Here's how the part is built. I have some questions about the finished solid (model axes, mm). Face numbers are marked on the shaded views. A direction names the side the tool comes from. Coordinates: 2 decimals unless noted, no trailing zeros. Write each loop counter-clockwise with the first axis right and the second up, starting at its lowest first coordinate (ties: lowest second). Pieces come first, ordered by that corner, then holes. Notation, with made-up numbers: M 2,-28 L 7,-28 A13 cw 7,-11 Z; hole C 85,-38.75 d6. An arc over 180 degrees is marked long. Use a Markdown table: item, result.
```python
from build123d import *

# Parameters (mm, degrees)
BOSS_EXTRUDE1_DEPTH = 30
SKETCH3_R           = 2
CUT_EXTRUDE1_DEPTH  = 49.344936653
FILLET1_R           = 2.5


with BuildPart() as part:
    # Sketch2 → Boss-Extrude1 (new, symmetric)
    with BuildSketch(Plane(origin=(0, 0, 0), x_dir=(0, 0, -1), z_dir=(1, 0, 0))):
        with BuildLine():
            Line((0, 0), (17.093183557, 0))
            ThreePointArc((17.093183557, 0), (23.540778857, 1.87930265), (27.968877001, 6.928580859))
            Line((27.968877001, 6.928580859), (32.531082361, 16.712261826))
            ThreePointArc((32.531082361, 16.712261826), (32.587511126, 16.763969262), (32.663974966, 16.760630779))
            Line((32.663974966, 16.760630779), (32.845236523, 16.676107126))
            ThreePointArc((32.845236523, 16.676107126), (33.879385242, 15.547531839), (33.812615574, 14.018255029))
            Line((33.812615574, 14.018255029), (30.053384911, 5.956558857))
            ThreePointArc((30.053384911, 5.956558857), (24.776567956, -0.060497675), (17.093183557, -2.3))
            Line((17.093183557, -2.3), (2.3, -2.3))
            Line((2.3, -2.3), (0, 0))
        make_face()
    extrude(amount=BOSS_EXTRUDE1_DEPTH, both=True)

    # Sketch3 → Cut-Extrude1 (cut, through all)
    with BuildSketch(Plane(origin=(0, 0, 0), x_dir=(1, 0, 0), z_dir=(0, 1, 0))):
        with BuildLine():
            Line((-26.9, 13.33), (-30, 13.33))
            Line((-30, 13.33), (-30, 0))
            Line((-30, 0), (-22.5, 0))
            Line((-22.5, 0), (-22.5, 8.93))
            ThreePointArc((-22.5, 8.93), (-23.788730163, 12.041269837), (-26.9, 13.33))
        make_face()
        with Locations(Location((-17, 9.5, 0), (0, 0, 270))):
            Circle(SKETCH3_R)
        with Locations(Location((17, 9.5, 0), (0, 0, 270))):
            Circle(SKETCH3_R)
        with BuildLine():
            Line((30, 0), (30, 13.33))
            Line((30, 13.33), (26.9, 13.33))
            ThreePointArc((26.9, 13.33), (23.788730163, 12.041269837), (22.5, 8.93))
            Line((22.5, 8.93), (22.5, 0))
            Line((22.5, 0), (30, 0))
        make_face()
    extrude(amount=-CUT_EXTRUDE1_DEPTH, mode=Mode.SUBTRACT)

    # Fillet1
    fillet1_edges = [part.edges().sort_by_distance(p)[0] for p in [
        (-30, -1.15, -13.33),
        (30, -1.15, -13.33),
    ]]
    fillet(fillet1_edges, radius=FILLET1_R)


solid = part.part
```
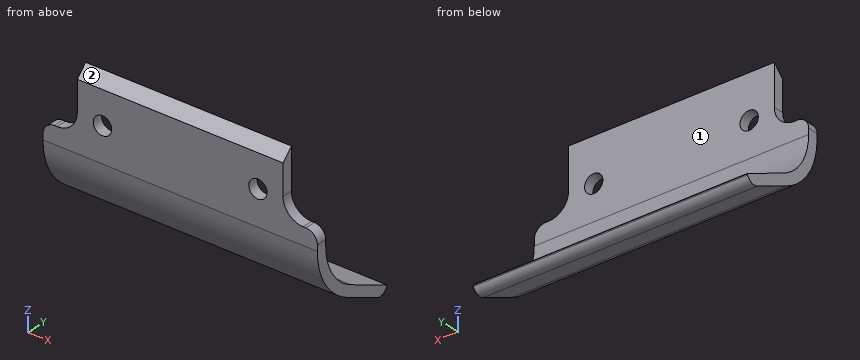
1. Suppose I cut it at A-A on x = 17. Write out the boundary of the cut face in (y, z).
Answers follow:
| item | result |
|---|---|
| outline | M -2.3,-17.09 A14.3 ccw 5.96,-30.05 L 14.02,-33.81 A2 ccw 16.68,-32.85 L 16.76,-32.66 A0.1 ccw 16.71,-32.53 L 6.93,-27.97 A12 cw 0,-17.09 L 0,-11.5 L -2.3,-11.5 Z; M -2.3,-7.5 L 0,-7.5 L 0,0 L -2.3,-2.3 Z |
2. Will these pins go through, and if not, where does the flat tip stop? pin 1 Ø8.5 at (x, z) = (-13.5, -10.5) entering from +Y; pin 2 Ø6 at (x, y) = (-15, 13.5) entering from +Z; pin 3 Ø1.8 at (y, z) = (-0.5, -2.5) entering from -X.
Answers follow:
| item | result |
|---|---|
| pin 1 | stops at y = 0 |
| pin 2 | stops at z = -29.63 |
| pin 3 | stops at x = -22.5 |
3. Suppose I cut it at D-D on z = -4. Write out the boundary of the cut face in (x, y).
Answers follow:
| item | result |
|---|---|
| outline | M -22.5,-2.3 L 22.5,-2.3 L 22.5,0 L -22.5,0 Z |
4. Which directions (+Z, -Z, +X, -X, +Y, -Y) give clear straight access to the entire face, cutting with the end or side of a thin tool? Please do the marked faces 1 and 2.
Answers follow:
| item | result |
|---|---|
| face 1 | +Z, +X, -X, +Y |
| face 2 | +Z, +X, -X, -Y |
5. Suppose I cut it at B-B on y = -1. Write out the boundary of the cut face in (x, z).
Answers follow:
| item | result |
|---|---|
| outline | M -30,-23.05 L 30,-23.05 L 30,-15.83 A2.5 ccw 27.5,-13.33 L 26.9,-13.33 A4.4 cw 22.5,-8.93 L 22.5,-1 L -22.5,-1 L -22.5,-8.93 A4.4 cw -26.9,-13.33 L -27.5,-13.33 A2.5 ccw -30,-15.83 Z; hole C -17,-9.5 d4; hole C 17,-9.5 d4 |
6. I need wall thicknesses on probe 1 along X at (y, z) = (-1.2, -9.5); probe 2 along Y at (x, z) = (6, -6); probe 3 along Y at (x, z) = (11, -20). Which ranges of each line are inside material? Lowest first, please.
Answers follow:
| item | result |
|---|---|
| probe 1 | x = -22.54 to -19, -15 to 15, 19 to 22.54 |
| probe 2 | y = -2.3 to 0 |
| probe 3 | y = -2 to 0.36 |
7. Suppose I cut it at C-C on x = 5. Write out the boundary of the cut face in (y, z).
Answers follow:
| item | result |
|---|---|
| outline | M -2.3,-17.09 A14.3 ccw 5.96,-30.05 L 14.02,-33.81 A2 ccw 16.68,-32.85 L 16.76,-32.66 A0.1 ccw 16.71,-32.53 L 6.93,-27.97 A12 cw 0,-17.09 L 0,0 L -2.3,-2.3 Z |
